Can you work these out from the drawing? Everything is in mm from the part's minimum corner. A direction names the side the tool comes from. Coordinates: 2 decimals unless noted, no trailing zeros. Write each loop counter-clockwise with the first axis right and the second up, starting at its lowest first coordinate (ties: lowest second). Pieces come first, ordered by that corner, then holes. Notation, with made-up numbers: M -18,-40 L 0,-40 A25 cw 0,-15 Z; hole C -37.75,-33.5 d10. An arc over 180 degrees is marked long. Answer as a JSON object with one key per item and string values. Group by question number.
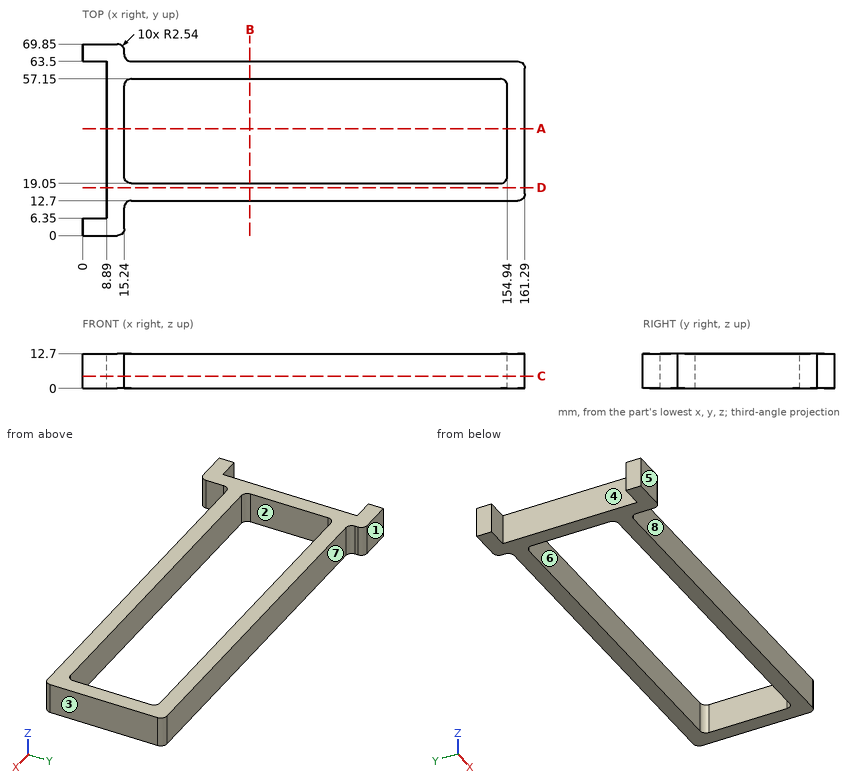
Q1. Will these pins go through, and if not, where does the flat tip stop? pin 1 (2 mm diameter, centred on y = 28, z = 1.5, fed in from -X); pin 2 (5 mm diameter, centred on y = 8.5, z = 3, fed in from +X); pin 3 (4 mm diameter, centred on y = 5.5, z = 8, fed in from +X).
Q2. We'd pull the mould along Y, two halves only. Please class the marked faces 1, 2, 3 and 4: pulls with the +Y half, pulls with the -Y half, needs draft (parallel to the pull), parting line crosses it, or undercut.
Q3. If we section it at A-A on y = 39: List the corners of the cut face in (x, z) for me.
Q4. On a 3-axis mill with a long thin cutter (end or side, diameter ignored), from which of +Z, -Z, +X, -X, +Y, -Y can I reach the whole of each face in a straight line? I mean the marked faces 5, 6, 7 and 8. Say none if no direction works.
Q5. If we section it at D-D on y = 17.5: List the corners of the cut face in (x, z) for me.
Q6. If we section it at B-B on x = 61: List the corners of the cut face in (y, z) for me.
Q7. Please list where these lines run through material, in increasing order: L1, parallel to X at y = 38, z = 8.5; L2, parallel to Y at x = 50.5, z = 3.5; L3, parallel to X at y = 4, z = 5.
Q8. If we section it at C-C on z = 4.5: List the corners of the cut face in (x, y) for me, and give its area (3 significant figures).
Reply:
{
 "1": {"pin 1": "x = 8.89", "pin 2": "x = 15.38", "pin 3": "x = 15.24"},
 "2": {"face 1": "pulls with the +Y half", "face 2": "undercut", "face 3": "needs draft", "face 4": "undercut"},
 "3": {"outline": "M 8.89,0 L 15.24,0 L 15.24,12.7 L 8.89,12.7 Z; M 154.94,0 L 161.29,0 L 161.29,12.7 L 154.94,12.7 Z"},
 "4": {"face 5": "+Z, -Z, +X, -X, -Y", "face 6": "+Z, -Z", "face 7": "+Z, -Z, +X, +Y", "face 8": "+Z, -Z, +X, -Y"},
 "5": {"outline": "M 8.89,0 L 161.29,0 L 161.29,12.7 L 8.89,12.7 Z"},
 "6": {"outline": "M 12.7,0 L 19.05,0 L 19.05,12.7 L 12.7,12.7 Z; M 57.15,0 L 63.5,0 L 63.5,12.7 L 57.15,12.7 Z"},
 "7": {"L1": "8.89 to 15.24, 154.94 to 161.29", "L2": "12.7 to 19.05, 57.15 to 63.5", "L3": "0 to 15.24"},
 "8": {"outline": "M 0,0 L 12.7,0 A2.54 ccw 15.24,2.54 L 15.24,10.16 A2.54 cw 17.78,12.7 L 158.75,12.7 A2.54 ccw 161.29,15.24 L 161.29,60.96 A2.54 ccw 158.75,63.5 L 17.78,63.5 A2.54 cw 15.24,66.04 L 15.24,67.31 A2.54 ccw 12.7,69.85 L 0,69.85 L 0,63.5 L 8.89,63.5 L 8.89,6.35 L 0,6.35 Z; hole M 15.24,21.59 A2.54 ccw 17.78,19.05 L 152.4,19.05 A2.54 ccw 154.94,21.59 L 154.94,54.61 A2.54 ccw 152.4,57.15 L 17.78,57.15 A2.54 ccw 15.24,54.61 Z", "area": "2,660 mm^2"}
}
